```python
from build123d import *

# Parameters (mm, degrees)
SKETCH1_W                          = 44
SKETCH1_H                          = 210
BASE_FLANGE1_DEPTH                 = 0.5
SKETCH6_R                          = 5
CUT_EXTRUDE1_DEPTH                 = 10
LPATTERN1_COUNT                    = 8
LPATTERN1_PITCH                    = 25
EDGE_FLANGE2_STRIP_W               = 3.4732
EDGE_FLANGE2_STRIP_H               = 0.5
EDGE_FLANGE2_STRIP_CUT_DEPTH       = 210
EDGE_FLANGE2_DEPTH                 = 210
F_7_0_7_DIAMETER_HOLE2_D           = 7
F_7_0_7_DIAMETER_HOLE2_DEPTH       = 60
F_7_0_7_DIAMETER_HOLE2_CSINK_D     = 7.05
F_7_0_7_DIAMETER_HOLE2_CSINK_ANGLE = 90
F_7_0_7_DIAMETER_HOLE2_TIP         = 2.103012167
BREAK_CORNER2_START                = 22
BREAK_CORNER2_DEPTH                = 0.5


# Read off the part's stored shape, not the designer's step: Break-Corner2
# Sheet-metal steps are written as plain solids
with BuildPart() as part:
    # Sketch1 → Base-Flange1 (new body)
    with BuildSketch(Plane.XY):
        Rectangle(SKETCH1_W, SKETCH1_H)
    extrude(amount=-BASE_FLANGE1_DEPTH)

    # Sketch6 → Cut-Extrude1 (cut)
    with BuildSketch(Plane.XY):
        with Locations((11, 95)):
            Circle(SKETCH6_R)
        with Locations((-10.650635095, 82.5)):
            Circle(SKETCH6_R)
    cut_extrude1 = extrude(amount=-CUT_EXTRUDE1_DEPTH, mode=Mode.SUBTRACT)

    # LPattern1: Cut-Extrude1 ×8
    with Locations(*[(0, -i * LPATTERN1_PITCH, 0) for i in range(1, LPATTERN1_COUNT)]):
        add(cut_extrude1, mode=Mode.SUBTRACT)

    # Edge-Flange2 strip (across the edge) → Edge-Flange2 strip cut (cut)
    with BuildSketch(Plane(origin=(22, -105, 0), x_dir=(-1, 0, 0), z_dir=(0, 1, 0))):
        with Locations((-1, -0.25)):
            Rectangle(EDGE_FLANGE2_STRIP_W, EDGE_FLANGE2_STRIP_H)
    extrude(amount=EDGE_FLANGE2_STRIP_CUT_DEPTH, mode=Mode.SUBTRACT)

    # Edge-Flange2 section (across the edge) → Edge-Flange2 (add)
    with BuildSketch(Plane(origin=(22, -105, 0), x_dir=(-1, 0, 0), z_dir=(0, 1, 0))):
        with BuildLine():
            Line((-0.5, 0.7366), (-0.5, 19.5))
            Line((-0.5, 19.5), (0, 19.5))
            Line((0, 19.5), (0, 0.7366))
            ThreePointArc((0, 0.7366), (0.215745145, 0.215745145), (0.7366, 0))
            Line((0.7366, 0), (0.7366, -0.5))
            ThreePointArc((0.7366, -0.5), (-0.137808246, -0.137808246), (-0.5, 0.7366))
        make_face()
    extrude(amount=EDGE_FLANGE2_DEPTH)

    # Ø7.0 (7) Diameter Hole2
    with Locations(Plane(origin=(22.5, 0, 0), x_dir=(0, 0, -1), z_dir=(1, 0, 0))):
        with Locations((-11.5, 95), (-11.5, -95)):
            CounterSinkHole(F_7_0_7_DIAMETER_HOLE2_D / 2, F_7_0_7_DIAMETER_HOLE2_CSINK_D / 2, depth=F_7_0_7_DIAMETER_HOLE2_DEPTH, counter_sink_angle=F_7_0_7_DIAMETER_HOLE2_CSINK_ANGLE)
            with Locations((0, 0, -(F_7_0_7_DIAMETER_HOLE2_DEPTH + F_7_0_7_DIAMETER_HOLE2_TIP / 2))):  # 118° drill point
                Cone(0, F_7_0_7_DIAMETER_HOLE2_D / 2, F_7_0_7_DIAMETER_HOLE2_TIP, mode=Mode.SUBTRACT)

    # Break-Corner2 outline → Break-Corner2 (cut)
    with BuildSketch(Plane.YZ.offset(BREAK_CORNER2_START)):
        Polygon((-105, 19.5), (-105, 17.5), (-103, 19.5), align=None)
        Polygon((105, 19.5), (103, 19.5), (105, 17.5), align=None)
    extrude(amount=BREAK_CORNER2_DEPTH, mode=Mode.SUBTRACT)


solid = part.part
```
Could you check a few things on this model? Use its own coordinates, in mm. A direction names the side the tool comes from. Coordinates: 2 decimals unless noted, no trailing zeros. Loops run counter-clockwise (first coordinate to the right, second up) from the corner with the lowest first, then second, coordinate; pieces in that order, holes last.
1) Thinking about a two-plate mould opening in X: for faces 3 (the face through (9.92, 90.12, -0.25)), 4 (the face through (-11.735, -22.381, -0.246)), 5 (the face through (22, -1, 10)), 6 (the face through (22.234, -98.417, 10.741)), which applies, released by +X, released by -X, zero draft, split by the parting line, or undercut?
Reported:
face 3: undercut
face 4: undercut
face 5: released by -X
face 6: zero draft
2) Imagine slicing it at B-B (y = 95). List the corners of the cut face in (x, z) for me (3 decimals).
Reported:
outline: (-22, -0.5) - (6, -0.5) - (6, 0) - (-22, 0) - close; (16, -0.5) - (21.263, -0.5) arc R1.237 ccw to (22.5, 0.737) - (22.5, 7.975) - (22.475, 8) - (22, 8) - (22, 0.737) arc R0.737 cw to (21.263, 0) - (16, 0) - close; (22, 15) - (22.475, 15) - (22.5, 15.025) - (22.5, 19.5) - (22, 19.5) - close
3) Which directions (+Z, -Z, +X, -X, +Y, -Y) give clear straight access to the entire face, cutting with the end or side of a thin tool? Please do faces 1 (the face through (-1, 1, 0)), 2 (the face through (-11.735, 27.619, -0.246)).
Reported:
face 1: +Z, -X, +Y, -Y
face 2: +Z, -Z
4) Imagine slicing it at D-D (x = 2). List the corners of the cut face in (y, z) for me, and give its area (3 significant figures).
Reported:
outline: (-105, -0.5) - (105, -0.5) - (105, 0) - (-105, 0) - close
area: 105 mm2
5) Imagine slicing it at C-C (x = 11). State how many separate pieces and enclosed holes the cut face has, and give its area (3 significant figures).
Reported:
separate pieces: 9
enclosed holes: 0
area: 65.0 mm2
6) Will these pins go through, and if not, where does the flat tip stop? pin 1 Ø11.5 at (x, y) = (11, -30) entering from +Z; pin 2 Ø10 at (y, z) = (-16.5, 10) entering from -X; pin 3 Ø9 at (x, y) = (11, 95) entering from +Z (3 decimals).
Reported:
pin 1: stops at z = 0
pin 2: stops at x = 22
pin 3: passes through
7) Please list where these lines run through material, in increasing order: line 1 along Z through (x, y) = (-19, -74); line 2 along X through (y, z) = (34, 7).
Reported:
line 1: z = -0.5 to 0
line 2: x = 22 to 22.5
8) Imagine slicing it at A-A (y = -42.5). List the corners of the cut face in (x, z) for me.
Reported:
outline: (-22, -0.5) - (-15.65, -0.5) - (-15.65, 0) - (-22, 0) - close; (-5.65, -0.5) - (21.26, -0.5) arc R1.24 ccw to (22.5, 0.74) - (22.5, 19.5) - (22, 19.5) - (22, 0.74) arc R0.74 cw to (21.26, 0) - (-5.65, 0) - close
